from build123d import *

# Parameters (mm, degrees)
BOSS_EXTRUDE1_DEPTH = 6.35


with BuildPart() as part:
    # Sketch1 → Boss-Extrude1 (new body)
    with BuildSketch(Plane(origin=(0, 0, 0), x_dir=(1, 0, 0), z_dir=(0, 1, 0))):
        with BuildLine():
            Line((0, 294.386), (0, 290.152666667))
            Line((0, 290.152666667), (6.35, 290.152666667))
            Line((6.35, 290.152666667), (6.35, 285.919333333))
            Line((6.35, 285.919333333), (0, 285.919333333))
            Line((0, 285.919333333), (0, 281.686))
            ThreePointArc((0, 281.686), (-199.182080765, 199.182080765), (-281.686, 0))
            Line((-281.686, 0), (-285.919333333, 0))
            Line((-285.919333333, 0), (-285.919333333, 6.35))
            Line((-285.919333333, 6.35), (-290.152666667, 6.35))
            Line((-290.152666667, 6.35), (-290.152666667, 0))
            Line((-290.152666667, 0), (-294.386, 0))
            ThreePointArc((-294.386, 0), (-208.162336886, 208.162336886), (0, 294.386))
        make_face()
    extrude(amount=BOSS_EXTRUDE1_DEPTH)


solid = part.part
Check sheet for the modelled part. Datum: model origin and axes. Units: mm. A direction names the side the tool comes from. Round coordinates to 2 decimals unless told otherwise and drop trailing zeros. Order: outer loops, then holes, each group sorted by start corner. A loop starts at its lowest first (then second) coordinate and runs counter-clockwise, first axis right, second up. Notation, with made-up numbers: M 53,36 L 108,36 A17 cw 108,46 Z; hole C 32,-23.5 d11. An arc over 180 degrees is marked long. One line per item, written item: value. Start each with the question number.
1. Section check B-B on z = -199.5. Enter the section's corners in (x, y).
2. Section check C-C on x = -236.5. Enter the section's corners in (y, z), and give its area (4 significant figures).
3. Scan lines: line 1 along Z through (x, y) = (-174.5, 4); line 2 along Z through (x, y) = (-185.5, 4.75); line 3 along X through (y, z) = (4.25, -143). Record each from-to range of solid material in increasing order.
4. Gauge pin test, flat ends, axial feed: P1, Ø1.5, axis at y = 4, z = -152.5, coming from the +X side; P2, Ø1.3, axis at y = 4.5, z = -292, coming from the +X side; P3, Ø1.9, axis at y = 2.5, z = -2, coming from the -X side. Record the tip position at first contact, or that the pin passes through.
5. Access from +Z, -Z, +X, -X, +Y, -Y to the whole of each face (thin tool, end or side, straight path). Record for faces 5 (the flat face through (3, 3, -285.919)), 6 (the flat face through (-188, 0, -213)).
6. Release check for a two-part mould opening along X. For faces 1 (the flat face through (-290.153, 3, -3)), 2 (the flat face through (-285.919, 3, -3)), 3 (the cylindrical face through (-196.98, 3.13, -201.36)), 4 (the flat face through (3, 3, -290.153)) record: released by +X, released by -X, zero draft, split by the parting line, or undercut.
7. Section check A-A on y = 2.5. Enter the section's corners in (x, z).
Results found:
1. outline: M -216.48,0 L -198.86,0 L -198.86,6.35 L -216.48,6.35 Z
2. outline: M 0,-175.3 L 6.35,-175.3 L 6.35,-153.02 L 0,-153.02 Z
2. area: 141.5 mm^2
3. line 1: -237.09 to -221.13
3. line 2: -228.59 to -211.98
3. line 3: -257.32 to -242.69
4. P1: x = -236.35
4. P2: x = 0
4. P3: x = -294.38
5. face 5: +Z, +X, +Y, -Y
5. face 6: +Z, -Z, +X, -X, -Y
6. face 1: undercut
6. face 2: undercut
6. face 3: released by +X
6. face 4: zero draft
7. outline: M -294.39,0 A294.39 ccw 0,-294.39 L 0,-290.15 L 6.35,-290.15 L 6.35,-285.92 L 0,-285.92 L 0,-281.69 A281.69 cw -281.69,0 L -285.92,0 L -285.92,-6.35 L -290.15,-6.35 L -290.15,0 Z
